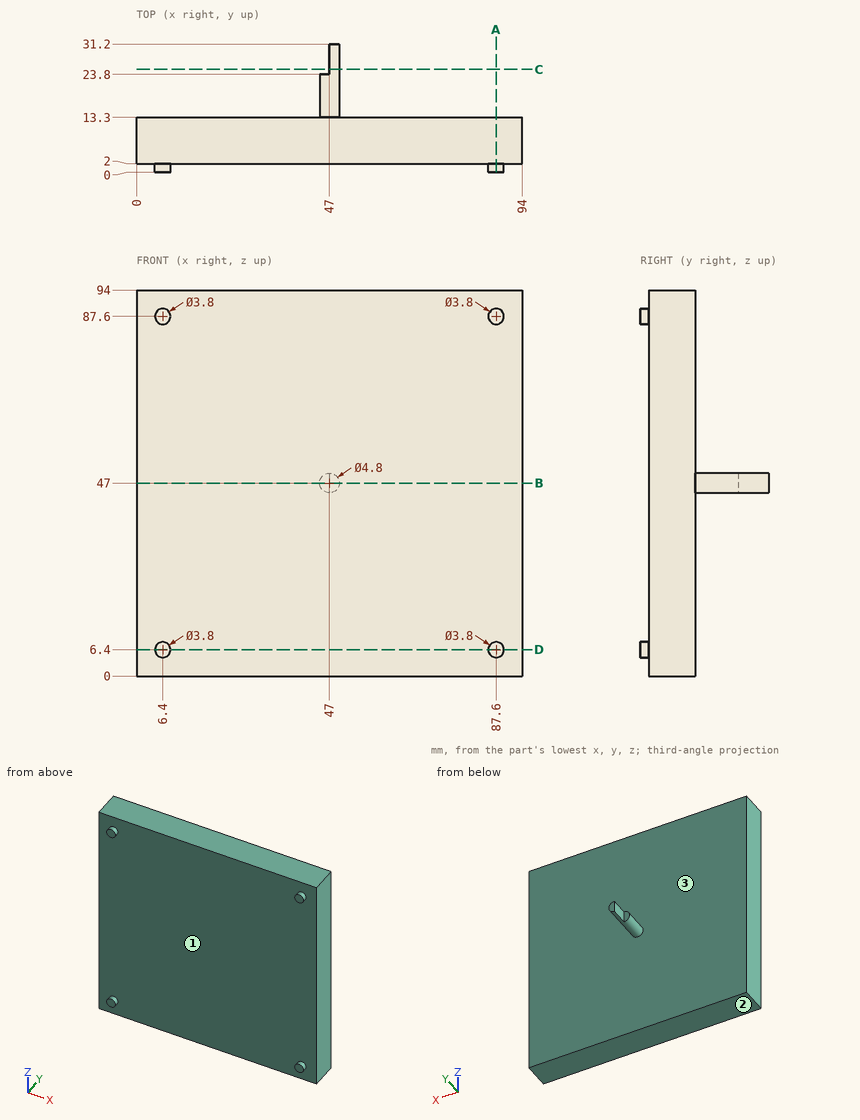
Print and shaded views of the part. All mm, measured from the part's lowest x, y and z. Round coordinates to 2 decimals unless told otherwise and drop trailing zeros. Write each loop counter-clockwise with the first axis right and the second up, starting at its lowest first coordinate (ties: lowest second). Pieces come first, ordered by that corner, then holes.
(1) Slice it at C-C, the plane y = 25. Write the cut outline in (x, z), and give its area (3 significant figures).
(2) Probe line 1 along Y through (x, z) = (26, 48); line 2 along Z through (x, y) = (46.5, 22.5); line 3 along X through (y, z) = (28.5, 49). List the from-to ranges inside material, lowest first.
(3) Mould opens along Y. For the marked faces 1, 2 and 3 say: pulls with the +Y half, pulls with the -Y half, needs draft (parallel to the pull), parting line crosses it, or undercut.
(4) Slice it at D-D, the plane z = 6.4. Write the cut outline in (x, y).
(5) Slice it at A-A, the plane x = 87.6. Write the cut outline in (y, z), and give its area (3 significant figures).
(6) Drop flat-ended pins along their axis: P1, Ø2.5, axis at x = 45.5, z = 46, coming from the +Y side; P2, Ø1.5, axis at x = 42.5, z = 17.5, coming from the +Y side; P3, Ø1.4, axis at y = 27, z = 46.5, coming from the -X side; P4, Ø6, axis at y = 20, z = 41.5, coming from the +X side. Give the stop position or say it passes through.
(7) Slice it at B-B, the plane z = 47. Write the cut outline in (x, y), and give its area (3 significant figures).
From the geometry:
1. outline: (47, 44.6) arc R2.4 ccw to (47, 49.4) - close
1. area: 9.05 mm2
2. line 1: y = 2 to 13.3
2. line 2: z = 44.65 to 49.35
2. line 3: x = 47 to 48.33
3. face 1: pulls with the -Y half
3. face 2: needs draft
3. face 3: pulls with the +Y half
4. outline: (0, 2) - (4.5, 2) - (4.5, 0) - (8.3, 0) - (8.3, 2) - (85.7, 2) - (85.7, 0) - (89.5, 0) - (89.5, 2) - (94, 2) - (94, 13.3) - (0, 13.3) - close
5. outline: (0, 4.5) - (2, 4.5) - (2, 0) - (13.3, 0) - (13.3, 94) - (2, 94) - (2, 89.5) - (0, 89.5) - (0, 85.7) - (2, 85.7) - (2, 8.3) - (0, 8.3) - close
5. area: 1,080 mm2
6. P1: stops at y = 23.8
6. P2: stops at y = 13.3
6. P3: stops at x = 47
6. P4: passes through
7. outline: (0, 2) - (94, 2) - (94, 13.3) - (49.4, 13.3) - (49.4, 31.2) - (47, 31.2) - (47, 23.8) - (44.6, 23.8) - (44.6, 13.3) - (0, 13.3) - close
7. area: 1,130 mm2
